from build123d import *

# Parameters (mm, degrees)
F1_DEPTH = 80
F3_DEPTH = 80
F4_W     = 70.0248382054
F4_H     = 52.043965552
F5_DEPTH = 25


with BuildPart() as f1:
    # F0 (on Front) → F1 (new body)
    with BuildSketch(Plane.XZ):
        Polygon((-16.1164440215, 55.6217506528), (-33.0398865044, 0), (0, 0), (0, 55.6217506528), align=None)
        Polygon((0, 55.6217506528), (0, 0), (33.0398865044, 0), (16.1164440215, 55.6217506528), align=None)
    extrude(amount=F1_DEPTH)

    # F2 (on face) → F3 (cut)
    with BuildSketch(Plane.XZ.offset(80)):
        Polygon((-13.7641547164, 52.7867953574), (-28.990626716, 2.7424246723), (29.1717245215, 2.7424246723), (13.9452525218, 52.7867953574), align=None)
    extrude(amount=-F3_DEPTH, mode=Mode.SUBTRACT)

    # F4 (on face) → F5 (cut)
    with BuildSketch(Plane(origin=(-30.2404161362, 0, 9.200931958), x_dir=(0, -1, 0), z_dir=(-0.9566974319, 0, 0.2910842211))):
        with Locations((39.3633369822, 19.0598971676)):
            Rectangle(F4_W, F4_H)
    extrude(amount=-F5_DEPTH, mode=Mode.SUBTRACT)


solid = f1.part
For this review, take the finished solid that the model builds, in its own axes (mm). A direction names the side the tool comes from. Give positions to 0.01 mm unless a question says otherwise; leave off trailing zeros. Loops run counter-clockwise (first coordinate to the right, second up) from the corner with the lowest first, then second, coordinate; pieces in that order, holes last.
Item 1: Take a section at D-D, the plane z = 40.5. State the section outline as (x, y) points, and give its area (3 significant figures).
Item 2: Take a section at A-A, the plane y = -10.5. State the section outline as (x, z) points.
Item 3: Take a section at B-B, the plane x = -9. State the section outline as (y, z) points, and give its area (3 significant figures).
Item 4: Draft analysis for pull direction X (two halves, no side actions). For faces 4 (the flat face through (-22.2, 0, 25.9)), 5 (the flat face through (24.697, -39.44, 27.422)), 6 (the flat face through (-15.7, -38.9, 51.9)), 7 (the flat face through (-14.01, -49.08, 51.98)), state which applies: +X half, -X half, draft (parallel to the pull), parting line (faces both ways), or undercut.
Item 5: For line 1 along Z through (x, y) = (10.5, -65.5); line 2 along Z through (x, y) = (-13, -10); line 3 along X through (y, z) = (-36.5, 41), list the stretches that pass through material, from the lowest coordinate up.
Item 6: Insertion check: pin 1 (2 mm diameter, centred on x = -1.5, y = -18.5, fed in from -Z); pin 2 (2 mm diameter, centred on y = -26, z = 42.5, fed in from -X); pin 3 (1 mm diameter, centred on y = -19.5, z = 49.5, fed in from +X); pin 4 (1 mm diameter, centred on y = -68.5, z = 22, fed in from -X). Each pin has a flat end and moves straight along its axis. Give the tip position at first contact, or say it passes through.
Item 7: Take a section at C-C, the plane x = 8.5. State the section outline as (y, z) points, and give its area (3 significant figures).
Item 8: Tool access review of faces 1 (the flat face through (13, -41, 2.742)), 2 (the flat face through (-24, -74.376, 21)), 3 (the flat face through (-28.151, -38.873, 1.288)): name each direction out of +Z, -Z, +X, -X, +Y, -Y from which nothing blocks a thin tool from reaching the whole face with its end or side.
Calculated:
1. outline: (-20.72, -80) - (-17.5, -80) - (-17.5, -74.38) - (-20.72, -74.38) - close; (-20.72, -4.35) - (-17.5, -4.35) - (-17.5, 0) - (-20.72, 0) - close; (17.68, -80) - (20.72, -80) - (20.72, 0) - (17.68, 0) - close
1. area: 275 mm2
2. outline: (-33.04, 0) - (-23.92, 0) - (-32.27, 2.54) - close; (-17.12, 52.33) - (-14.18, 51.44) - (-13.76, 52.79) - (13.95, 52.79) - (29.17, 2.74) - (-6.07, 2.74) - (-6.91, 0) - (33.04, 0) - (16.12, 55.62) - (-16.12, 55.62) - close
3. outline: (-80, 0) - (-74.38, 0) - (-74.38, 2.74) - (-80, 2.74) - close; (-80, 52.79) - (0, 52.79) - (0, 55.62) - (-80, 55.62) - close; (-4.35, 0) - (0, 0) - (0, 2.74) - (-4.35, 2.74) - close
3. area: 254 mm2
4. face 4: draft
4. face 5: +X half
4. face 6: -X half
4. face 7: undercut
5. line 1: z = 0 to 2.74, 52.79 to 55.62
5. line 2: z = 52.79 to 55.62
5. line 3: x = 17.53 to 20.57
6. pin 1: stops at z = 0
6. pin 2: stops at x = 16.77
6. pin 3: stops at x = 18.13
6. pin 4: stops at x = 23.16
7. outline: (-80, 0) - (0, 0) - (0, 2.74) - (-80, 2.74) - close; (-80, 52.79) - (0, 52.79) - (0, 55.62) - (-80, 55.62) - close
7. area: 446 mm2
8. face 1: +Y, -Y
8. face 2: none
8. face 3: +Z
